from build123d import *

# Parameters (mm, degrees)
BOSS_EXTRUDE1_START = -5
SKETCH1_R           = 2
BOSS_EXTRUDE1_DEPTH = 5


with BuildPart() as part:
    # Sketch1 → Boss-Extrude1 (new body)
    with BuildSketch(Plane.XY.offset(BOSS_EXTRUDE1_START)):
        with BuildLine():
            Line((-74.811187919, 158.283111414), (-22.442309188, 39.297815934))
            ThreePointArc((-22.442309188, 39.297815934), (-25.004479063, 32.707270772), (-31.595024225, 35.269440647))
            Line((-31.595024225, 35.269440647), (-83.963902956, 154.254736127))
            ThreePointArc((-83.963902956, 154.254736127), (-81.401733081, 160.845281289), (-74.811187919, 158.283111414))
        make_face()
        with Locations((-79.387545438, 156.26892377)):
            Circle(SKETCH1_R, mode=Mode.SUBTRACT)
        with Locations((-27.018666706, 37.283628291)):
            Circle(SKETCH1_R, mode=Mode.SUBTRACT)
    extrude(amount=-BOSS_EXTRUDE1_DEPTH)


solid = part.part
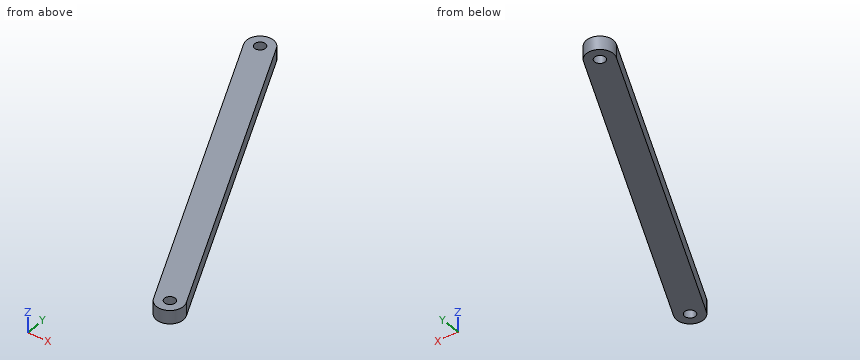
Geometry: final body of the model. Coordinates: model frame, mm. Give positions to 0.01 mm unless a question says otherwise; leave off trailing zeros. Loops run counter-clockwise (first coordinate to the right, second up) from the corner with the lowest first, then second, coordinate; pieces in that order, holes last. Notation, with made-up numbers: (-3, 52.25) -> (28, 52.25) arc R32 cw to (28, 86.25) -> close; hole circle Ø1 at (24.5, 26). An arc over 180 degrees is marked (long way). Put each result on its own line as item: value.
1. Ray query, line 1 along Y through (x, z) = (-27, -8.75); line 2 along Y through (x, z) = (-26, -8.95); line 3 along X through (y, z) = (83, -6.65). Return the intervals inside material, ascending. Write a range as [from, to].
Taken from the geometry:
line 1: y = [32.28, 35.28], [39.28, 49.65]
line 2: y = [32.39, 35.56], [39, 47.38]
line 3: x = [-52.6, -41.68]
2. Cut plane C-C (x = -71). Return the cut outline in (y, z).
Taken from the geometry:
outline: (124.8, -10) -> (149.62, -10) -> (149.62, -5) -> (124.8, -5) -> close
3. Cut plane A-A (z = -6.55). Return the cut outline in (x, y).
Taken from the geometry:
outline: (-83.96, 154.25) -> (-31.6, 35.27) arc R5 ccw to (-22.44, 39.3) -> (-74.81, 158.28) arc R5 ccw to start; hole circle Ø4 at (-79.39, 156.27); hole circle Ø4 at (-27.02, 37.28)
4. Cut plane B-B (y = 61). Return the cut outline in (x, z).
Taken from the geometry:
outline: (-42.92, -10) -> (-31.99, -10) -> (-31.99, -5) -> (-42.92, -5) -> close
5. Pin query (flat end, axial travel): P1, Ø1, axis at y = 146, z = -5.5, coming from the +X side; P2, Ø3, axis at x = -71, z = -8.5, coming from the +Y side; P3, Ø2, axis at y = 134.5, z = -8.5, coming from the -X side. Return the tip coordinate at first contact, or that it passes through.
Taken from the geometry:
P1: stops at x = -69.18
P2: stops at y = 153.03
P3: stops at x = -75.71
